Part model, mm, in its own coordinate system. Face numbers are marked on the shaded views. A direction names the side the tool comes from. Round coordinates to 2 decimals unless told otherwise and drop trailing zeros. Order: outer loops, then holes, each group sorted by start corner. A loop starts at its lowest first (then second) coordinate and runs counter-clockwise, first axis right, second up. Notation, with made-up numbers: (-3.5, 55.25) -> (50.5, 55.25) arc R16 cw to (50.5, 61.25) -> close; hole circle Ø1 at (-3, -19). An arc over 180 degrees is marked (long way). Return JSON: item names as keys, results as strings. Group by question number.
from build123d import *

# Parameters (mm, degrees)
F0_W      = 38
F0_H      = 38
F0_R      = 13
F1_DEPTH  = 2.8
F2_R      = 1.5
F3_DEPTH  = 2
F4_R      = 1
F5_DEPTH  = 1.5
F6_R      = 14.5
F6_R_2    = 13
F7_DEPTH  = 2
F9_DEPTH  = 2
F11_DEPTH = 17
F12_R     = 32
F12_R_2   = 13
F13_DEPTH = 2
F14_R     = 2.5
F15_DEPTH = 10
F18_R     = 10


with BuildPart() as f1:
    # F0 (on Right) → F1 (new body)
    with BuildSketch(Plane.YZ):
        Rectangle(F0_W, F0_H)
        Circle(F0_R, mode=Mode.SUBTRACT)
    extrude(amount=F1_DEPTH)

    # F2 (on face) → F3 (cut)
    with BuildSketch(Plane.YZ.offset(2.8)):
        with Locations((16.25, -7.5)):
            Circle(F2_R)
        with BuildLine():
            ThreePointArc((-14.75, -7.5), (-17.3106601718, -6.4393398282), (-16.25, -9))
            ThreePointArc((-16.25, -9), (-15.1893398282, -8.5606601718), (-14.75, -7.5))
        make_face()
        with Locations((16.25, 7.5)):
            Circle(F2_R)
        with BuildLine():
            ThreePointArc((-6, -16.25), (-7.5, -14.75), (-9, -16.25))
            ThreePointArc((-9, -16.25), (-7.5, -17.75), (-6, -16.25))
        make_face()
        with Locations((7.5, -16.25)):
            Circle(F2_R)
        with Locations((7.5, 16.25)):
            Circle(F2_R)
        with Locations((-16.25, 7.5)):
            Circle(F2_R)
        with Locations((-7.5, 16.25)):
            Circle(F2_R)
    extrude(amount=-F3_DEPTH, mode=Mode.SUBTRACT)

    # F4 (on face) → F5 (cut)
    with BuildSketch(Plane(origin=(0, 0, 0), x_dir=(0, -1, 0), z_dir=(-1, 0, 0))):
        with BuildLine():
            ThreePointArc((-15.25, -7.5), (-16.9571067812, -6.7928932188), (-16.25, -8.5))
            ThreePointArc((-16.25, -8.5), (-15.5428932188, -8.2071067812), (-15.25, -7.5))
        make_face()
        with BuildLine():
            ThreePointArc((-6.5, -16.25), (-7.5, -15.25), (-8.5, -16.25))
            ThreePointArc((-8.5, -16.25), (-7.5, -17.25), (-6.5, -16.25))
        make_face()
        with Locations((-16.25, 7.5)):
            Circle(F4_R)
        with Locations((-7.5, 16.25)):
            Circle(F4_R)
        with Locations((7.5, 16.25)):
            Circle(F4_R)
        with Locations((7.5, -16.25)):
            Circle(F4_R)
        with Locations((16.25, -7.5)):
            Circle(F4_R)
        with Locations((16.25, 7.5)):
            Circle(F4_R)
    extrude(amount=-F5_DEPTH, mode=Mode.SUBTRACT)

    # F6 (on face) → F7 (join)
    with BuildSketch(Plane(origin=(0, 0, 0), x_dir=(0, -1, 0), z_dir=(-1, 0, 0))):
        Circle(F6_R)
        Circle(F6_R_2, mode=Mode.SUBTRACT)
    extrude(amount=F7_DEPTH)

    # F8 (on face) → F9 (join)
    with BuildSketch(Plane(origin=(-2, 0, 0), x_dir=(0, -1, 0), z_dir=(-1, 0, 0))):
        with BuildLine():
            Line((-13, 0), (-14.5, 0))
            ThreePointArc((-14.5, 0), (0, -14.5), (14.5, 0))
            Line((14.5, 0), (13, 0))
            ThreePointArc((13, 0), (0, -13), (-13, 0))
        make_face()
        with BuildLine():
            Line((-14.5, 0), (-32, 0))
            ThreePointArc((-32, 0), (0, -32), (32, 0))
            Line((32, 0), (14.5, 0))
            ThreePointArc((14.5, 0), (0, -14.5), (-14.5, 0))
        make_face()
    extrude(amount=F9_DEPTH)

    # F10 (on face) → F11 (join)
    with BuildSketch(Plane(origin=(-4, 0, 0), x_dir=(0, -1, 0), z_dir=(-1, 0, 0))):
        with BuildLine():
            Line((-30, 0), (-32, 0))
            ThreePointArc((-32, 0), (0, -32), (32, 0))
            Line((32, 0), (30, 0))
            ThreePointArc((30, 0), (0, -30), (-30, 0))
        make_face()
    extrude(amount=F11_DEPTH)

    # F12 (on face) → F13 (join)
    with BuildSketch(Plane(origin=(-21, 0, 0), x_dir=(0, -1, 0), z_dir=(-1, 0, 0))):
        Circle(F12_R)
        Circle(F12_R_2, mode=Mode.SUBTRACT)
    extrude(amount=F13_DEPTH)

    # F14 (on face) → F15 (cut)
    with BuildSketch(Plane(origin=(-23, 0, 0), x_dir=(0, -1, 0), z_dir=(-1, 0, 0))):
        with BuildLine():
            ThreePointArc((-5, -16.25), (-7.5, -13.75), (-10, -16.25))
            ThreePointArc((-10, -16.25), (-7.5, -18.75), (-5, -16.25))
        make_face()
        with BuildLine():
            ThreePointArc((-13.75, -7.5), (-18.017766953, -5.732233047), (-16.25, -10))
            ThreePointArc((-16.25, -10), (-14.482233047, -9.267766953), (-13.75, -7.5))
        make_face()
        with Locations((7.5, -16.25)):
            Circle(F14_R)
        with Locations((16.25, -7.5)):
            Circle(F14_R)
        with Locations((-16.25, 7.5)):
            Circle(F14_R)
        with Locations((16.25, 7.5)):
            Circle(F14_R)
        with Locations((7.5, 16.25)):
            Circle(F14_R)
        with Locations((-7.5, 16.25)):
            Circle(F14_R)
    extrude(amount=-F15_DEPTH, mode=Mode.SUBTRACT)

    # F16 (on Front) → F17 (revolve)
    with BuildSketch(Plane.XZ):
        Polygon((-23, -14.5), (-23, -13), (-27, -14.5), (-27, -16), align=None)
    revolve(axis=Axis((-14.0123711899, 0, 0), (-1, 0, 0)))

    # F18
    f18_edges = [f1.edges().sort_by_distance(p)[0] for p in [
        (1.4, 19, 19),
        (1.4, 19, -19),
        (1.4, -19, -19),
        (1.4, -19, 19),
    ]]
    fillet(f18_edges, radius=F18_R)


solid = f1.part
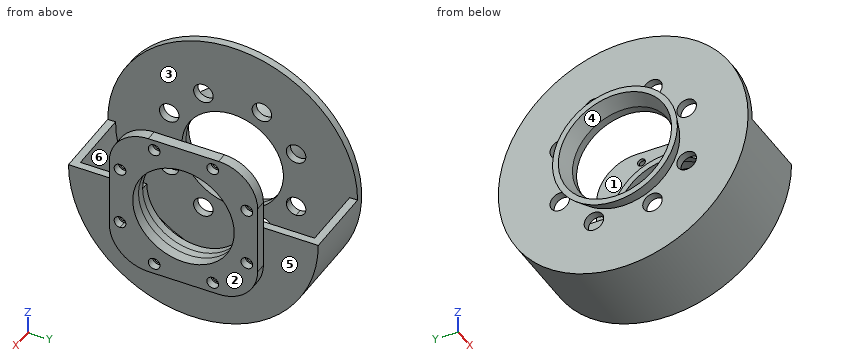
(1) Saw through at B-B, the plane x = -9. List the corners of the cut face in (y, z), and give its area (3 significant figures).
(2) Pin check, flat tips, straight feed: P1, Ø1.8, axis at y = 16.25, z = -7.5, coming from the -X side; P2, Ø1, axis at y = 20, z = 23.5, coming from the -X side; P3, Ø6, axis at x = -12, z = -6, coming from the +Y side; P4, Ø1.6, axis at y = -7.5, z = 16.25, coming from the -X side. Stop position of each tip, or through.
(3) Mould opens along Z. For the marked faces 4, 5 and 6 say: pulls with the +Z half, pulls with the -Z half, needs draft (parallel to the pull), parting line crosses it, or undercut.
(4) Tool access for the marked faces 1, 2 and 3: list every direction of +Z, -Z, +X, -X, +Y, -Y with a clear straight run to the whole face (end or side of a thin tool).
(5) Probe L1, parallel to X at y = -18, z = -4.5; L2, parallel to X at y = -23, z = -18; L3, parallel to Z at x = 2.05, y = -7.5. List the from-to ranges inside material, lowest first. Write a range as [from, to].
(6) Saw through at A-A, the plane z = -23. List the corners of the cut face in (x, y).
(7) Saw through at C-C, the plane y = -7.5. State how many separate pieces and enclosed holes the cut face has, and give its area (3 significant figures).
Results are:
{
 "1": {"outline": "(-32, 0) arc R32 ccw to (32, 0) -> (30, 0) arc R30 cw to (-30, 0) -> close", "area": "195 mm^2"},
 "2": {"P1": "stops at x = -4", "P2": "stops at x = -23", "P3": "stops at y = 31.86", "P4": "passes through"},
 "3": {"face 4": "undercut", "face 5": "needs draft", "face 6": "pulls with the +Z half"},
 "4": {"face 1": "none", "face 2": "+Z, -Z, +X, +Y, -Y", "face 3": "+Z"},
 "5": {"L1": "x = [-23, -21], [-4, -2], [0, 2.8]", "L2": "x = [-23, -21], [-4, -2]", "L3": "z = [-19, -17.75], [-14.75, -10.62], [10.62, 14.75], [17.75, 19]"},
 "6": {"outline": "(-23, -22.25) -> (-2, -22.25) -> (-2, 22.25) -> (-23, 22.25) -> close; hole (-21, -19.26) -> (-4, -19.26) -> (-4, 19.26) -> (-21, 19.26) -> close"},
 "7": {"separate pieces": "7", "enclosed holes": "0", "area": "191 mm^2"}
}
